The model under review builds one solid part; all positions refer to its coordinate system, in mm. A direction names the side the tool comes from. Coordinates: 2 decimals unless noted, no trailing zeros. Loops run counter-clockwise (first coordinate to the right, second up) from the corner with the lowest first, then second, coordinate; pieces in that order, holes last. Notation, with made-up numbers: M -25.5,-20 L 19.5,-20 A20 ccw 19.5,-13 Z; hole C 51,-4.75 d10. An arc over 180 degrees is marked long. Return JSON: item names as keys, results as strings.
```python
from build123d import *

# Parameters (mm, degrees)
ESQUISSE1_W             = 130
ESQUISSE1_H             = 70
BOSS_EXTRU_1_DEPTH      = 10
ENL_V_MAT_EXTRU_1_DEPTH = 2
ESQUISSE19_R            = 2
ENL_V_MAT_EXTRU_2_DEPTH = 20
ENL_V_MAT_EXTRU_3_DEPTH = 5


with BuildPart() as part:
    # Esquisse1 → Boss.-Extru.1 (new body)
    with BuildSketch(Plane.XY):
        with Locations((65, 35)):
            Rectangle(ESQUISSE1_W, ESQUISSE1_H)
    extrude(amount=BOSS_EXTRU_1_DEPTH)

    # Esquisse18 → Enlèv. mat.-Extru.1 (cut)
    with BuildSketch(Plane.XY.offset(10)):
        with BuildLine():
            Line((10, 5), (120, 5))
            ThreePointArc((120, 5), (123.535533906, 6.464466094), (125, 10))
            Line((125, 10), (125, 60))
            ThreePointArc((125, 60), (123.535533906, 63.535533906), (120, 65))
            Line((120, 65), (10, 65))
            ThreePointArc((10, 65), (6.464466094, 63.535533906), (5, 60))
            Line((5, 60), (5, 10))
            ThreePointArc((5, 10), (6.464466094, 6.464466094), (10, 5))
        make_face()
    extrude(amount=-ENL_V_MAT_EXTRU_1_DEPTH, mode=Mode.SUBTRACT)

    # Esquisse19 → Enlèv. mat.-Extru.2 (cut)
    with BuildSketch(Plane.ZY):
        with Locations((5, 56)):
            Circle(ESQUISSE19_R)
        with Locations((5, 14)):
            Circle(ESQUISSE19_R)
    extrude(amount=-ENL_V_MAT_EXTRU_2_DEPTH, mode=Mode.SUBTRACT)

    # Esquisse20 → Enlèv. mat.-Extru.3 (cut)
    with BuildSketch(Plane.XY.offset(8)):
        Polygon((10.050143374, 58), (110.050143374, 58), (110.050143374, 46), (14.191824128, 46), (14.191824128, 42), (110.050143374, 42), (110.050143374, 28), (14.191824128, 28), (14.191824128, 24), (110.050143374, 24), (110.050143374, 12), (10.050143374, 12), (10.050143374, 16), (106.050143374, 16), (106.050143374, 20), (10.191824128, 20), (10.191824128, 32), (106.050143374, 32), (106.050143374, 38.512028665), (10.191824128, 38.512028665), (10.191824128, 50), (106.050143374, 50), (106.050143374, 54), (10.050143374, 54), align=None)
    extrude(amount=-ENL_V_MAT_EXTRU_3_DEPTH, mode=Mode.SUBTRACT)


solid = part.part
```
1. Machinability: for faces 1 (the face through (0, 35, 5)), 2 (the face through (57, 50, 6)), which of the approach directions +Z, -Z, +X, -X, +Y, -Y give a long, thin tool a straight path to every point of the face, cutting with its end or side? Answer none if there is none.
Check values:
{"face 1": "+Z, -Z, -X, +Y, -Y", "face 2": "+Z"}
2. Add section A-A on y = 30. Give the boundary of the cut face in (x, z).
Check values:
{"outline": "M 0,0 L 130,0 L 130,10 L 125,10 L 125,8 L 110.05,8 L 110.05,3 L 10.19,3 L 10.19,8 L 5,8 L 5,10 L 0,10 Z"}
3. The part is to be moulded in two halves that separate along Y. For faces 3 (the face through (64, 35, 0)), 4 (the face through (64, 70, 5)), 5 (the face through (110.05, 35, 6)), say which applies: released by +Y, released by -Y, zero draft, split by the parting line, or undercut.
Check values:
{"face 3": "zero draft", "face 4": "released by +Y", "face 5": "undercut"}
4. To check wall thickness, follow line 1 (Y direction, x = 4.25, z = 5); line 2 (X direction, y = 17.5, z = 6.5); line 3 (Y direction, x = 20.5, z = 9). State the ranges of each line that lie inside material, in increasing order.
Check values:
{"line 1": "0 to 12, 16 to 54, 58 to 70", "line 2": "0 to 106.05, 110.05 to 130", "line 3": "0 to 5, 65 to 70"}
5. Add section C-C on y = 7.5. Give the boundary of the cut face in (x, z).
Check values:
{"outline": "M 0,0 L 130,0 L 130,10 L 124.33,10 L 124.33,8 L 5.67,8 L 5.67,10 L 0,10 Z"}
6. Insertion check: pin 1 Ø1.2 at (y, z) = (26, 6) entering from -X; pin 2 Ø1 at (x, y) = (70, 63) entering from +Z. Each pin has a flat end and moves straight along its axis. Give the tip position at first contact, or say it passes through.
Check values:
{"pin 1": "x = 0", "pin 2": "z = 8"}
